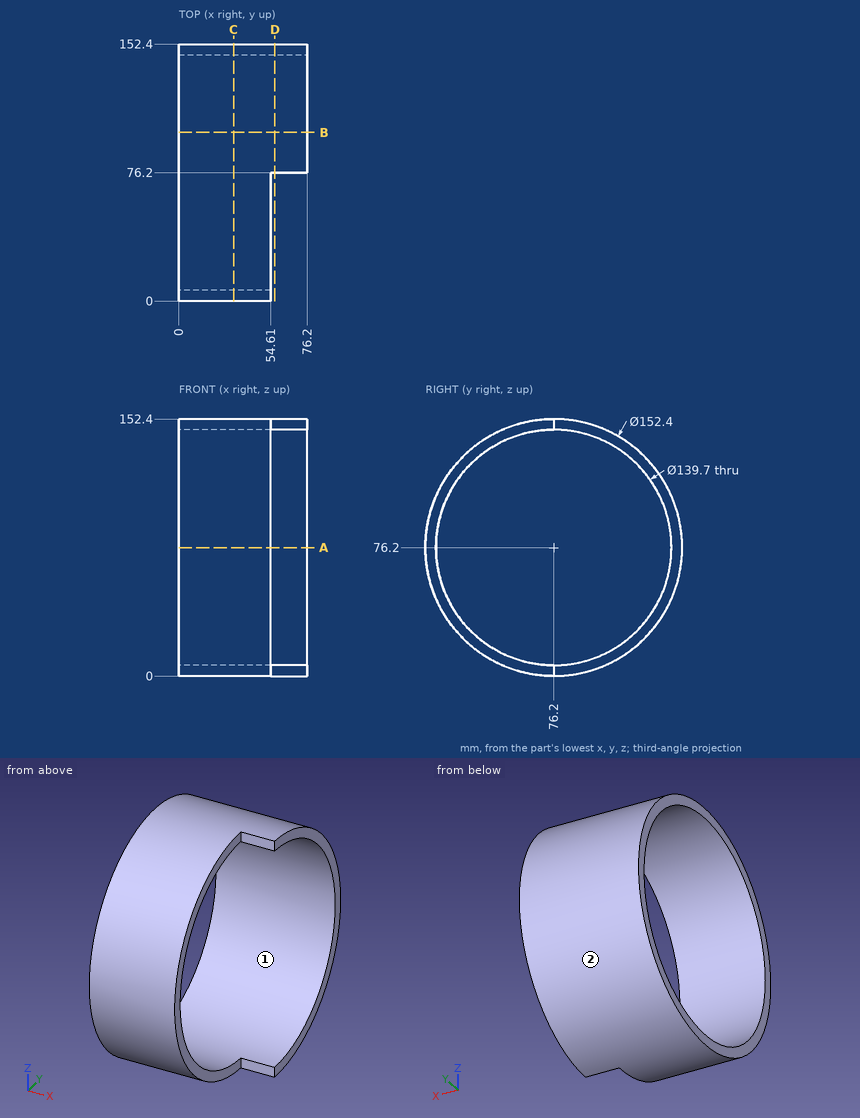
Source: three-view drawing plus pictorial views. Frame: mm from the lowest corner of the part. Round coordinates to 2 decimals unless told otherwise and drop trailing zeros. Order: outer loops, then holes, each group sorted by start corner. A loop starts at its lowest first (then second) coordinate and runs counter-clockwise, first axis right, second up. Notation, with made-up numbers: (52, 61) - (59, 61) arc R18 cw to (59, 75) - close; hole circle Ø8 at (3.5, 60.5). An arc over 180 degrees is marked (long way). Use a Markdown table: item, result.
1. First-contact query: pin 1 (3 mm diameter, centred on x = 61, z = 3.5, fed in from -Y); pin 2 (1.5 mm diameter, centred on x = 20, y = 83.5, fed in from -Z); pin 3 (5 mm diameter, centred on x = 27, z = 60, fed in from +Y). Flat tips, straight axial feed; report the tip coordinate or a pass-through.
Evaluation:
| item | result |
|---|---|
| pin 1 | y = 76.2 |
| pin 2 | z = 0.28 |
| pin 3 | y = 151.16 |
2. Section C-C on x = 32.5. Return the cut outline in (y, z).
Evaluation:
| item | result |
|---|---|
| outline | circle Ø152.4 at (76.2, 76.2); hole circle Ø139.7 at (76.2, 76.2) |
3. Material intervals for probe 1 along Z at (x, y) = (33, 76); probe 2 along Z at (x, y) = (55, 137.5), sorted ascending.
Evaluation:
| item | result |
|---|---|
| probe 1 | 0 to 6.35, 146.05 to 152.4 |
| probe 2 | 30.94 to 42.71, 109.69 to 121.46 |
4. Mould query, pull axis Z, two halves, no side actions, for the marked faces 1 and 2. Classes: +Z half, -Z half, draft (parallel to the pull), parting line (faces both ways), or undercut.
Evaluation:
| item | result |
|---|---|
| face 1 | undercut |
| face 2 | parting line |
5. Section D-D on x = 57. Return the cut outline in (y, z), then the cut area to 3 significant figures.
Evaluation:
| item | result |
|---|---|
| outline | (76.2, 0) arc R76.2 ccw to (76.2, 152.4) - (76.2, 146.05) arc R69.85 cw to (76.2, 6.35) - close |
| area | 1,460 mm^2 |
6. Section A-A on z = 76.2. Return the cut outline in (x, y), then the cut area to 3 significant figures.
Evaluation:
| item | result |
|---|---|
| outline | (0, 0) - (54.61, 0) - (54.61, 6.35) - (0, 6.35) - close; (0, 146.05) - (76.2, 146.05) - (76.2, 152.4) - (0, 152.4) - close |
| area | 831 mm^2 |
7. Section B-B on y = 100. Return the cut outline in (x, z), then the cut area to 3 significant figures.
Evaluation:
| item | result |
|---|---|
| outline | (0, 3.81) - (76.2, 3.81) - (76.2, 10.53) - (0, 10.53) - close; (0, 141.87) - (76.2, 141.87) - (76.2, 148.59) - (0, 148.59) - close |
| area | 1,020 mm^2 |
